from build123d import *

# Parameters (mm, degrees)
SKETCH2_R                       = 9.525
BOSS_EXTRUDE1_DEPTH             = 12.7
BOSS_EXTRUDE1_DIRECTION_2_REACH = 535.4


with BuildPart() as part:
    # Sketch1 → Revolve1 (revolve)
    with BuildSketch(Plane.XY):
        with BuildLine():
            Line((87.63, 445.77), (87.63, 87.63))
            ThreePointArc((87.63, 87.63), (61.963767, 25.666233), (0, 0))
            Line((0, 0), (0, 3.175))
            ThreePointArc((0, 3.175), (59.718703, 27.911297), (84.455, 87.63))
            Line((84.455, 87.63), (84.455, 445.77))
            ThreePointArc((84.455, 445.77), (59.718703, 505.488703), (0, 530.225))
            Line((0, 530.225), (0, 533.4))
            ThreePointArc((0, 533.4), (61.963767, 507.733767), (87.63, 445.77))
        make_face()
    revolve(axis=Axis((0, 533.4, 0), (0, 1, 0)))

    # Sketch2 → Boss-Extrude1 (add)
    with BuildSketch(Plane(origin=(0, 533.4, 0), x_dir=(1, 0, 0), z_dir=(0, 1, 0))):
        Circle(SKETCH2_R)
    extrude(amount=BOSS_EXTRUDE1_DEPTH)

    # Sketch2 → Boss-Extrude1 direction 2 (add, up to next)
    with BuildSketch(Plane(origin=(0, 533.4, 0), x_dir=(1, 0, 0), z_dir=(0, 1, 0)), mode=Mode.PRIVATE) as boss_extrude1_direction_2_sk1:
        Circle(SKETCH2_R)
    boss_extrude1_direction_2_tool1 = extrude(boss_extrude1_direction_2_sk1.sketch, amount=-BOSS_EXTRUDE1_DIRECTION_2_REACH, mode=Mode.PRIVATE) - part.part
    add(boss_extrude1_direction_2_tool1.solids().sort_by_distance((0, 533.4, 0))[0])


solid = part.part
Model file for the job. Use its own axes, mm. Coordinates: 2 decimals unless noted, no trailing zeros. Write each loop counter-clockwise with the first axis right and the second up, starting at its lowest first coordinate (ties: lowest second). Pieces come first, ordered by that corner, then holes. Notation, with made-up numbers: (-11.75, 28.25) -> (34.25, 28.25) arc R33 cw to (34.25, 57.25) -> close; hole circle Ø5 at (-1, -11). An arc over 180 degrees is marked (long way). One line per item, written item: value. Start each with the question number.
1) Slice it at A-A on y = 352.5. Write the cut outline in (x, z) (3 decimals).
2) Flat gauge pins, fed straight in: pin 1 Ø3 at (x, z) = (-50, 6.5) entering from +Y; pin 2 Ø1.5 at (y, z) = (271, 70) entering from -X; pin 3 Ø1.5 at (x, y) = (-65, 280) entering from -Z. Where does each tip first touch, or does it go through?
3) Pull direction X, two halves, no side cores. Call faces 1 (the face through (-18.996, 264.193, 85.546)), 2 (the face through (0, 546.1, 0)), 3 (the face through (38.971, 269.207, 74.926)): +X half, -X half, draft (parallel to the pull), parting line (faces both ways), or undercut.
4) Probe probe 1 along X at (y, z) = (334, 0) (3 decimals); probe 2 along Y at (x, z) = (-18, 56). List the from-to ranges inside material, lowest first.
Answers follow:
1. outline: circle Ø175.26 at (0, 0); hole circle Ø168.91 at (0, 0)
2. pin 1: y = 518.47
2. pin 2: x = -53.7
2. pin 3: z = -59.59
3. face 1: parting line
3. face 2: draft
3. face 3: undercut
4. probe 1: -87.63 to -84.455, 84.455 to 87.63
4. probe 2: 22.68 to 27.03, 506.37 to 510.72
